from build123d import *

# Parameters (mm, degrees)
SKETCH1_W           = 1
SKETCH1_H           = 18.5735
SKETCH2_R           = 0.7835
BOSS_EXTRUDE1_DEPTH = 0.2165
BOSS_EXTRUDE1_TAPER = -45
SKETCH3_R           = 1
BOSS_EXTRUDE2_DEPTH = 0.222374751
SKETCH4_R           = 1
BOSS_EXTRUDE3_DEPTH = 0.867625249
BOSS_EXTRUDE3_TAPER = -46.049277384
SKETCH5_R           = 1.9
BOSS_EXTRUDE4_DEPTH = 0.12
CUT_EXTRUDE1_DEPTH  = 0.9
CUT_EXTRUDE1_TAPER  = 15
CHAMFER1_SIZE       = 0.2165
FILLET1_R           = 0.5
SCALE1_SCALE        = 3.125


with BuildPart() as part:
    # Sketch1 → Revolve1 (revolve)
    with BuildSketch(Plane.XZ):
        with Locations((0.5, 10.71325)):
            Rectangle(SKETCH1_W, SKETCH1_H)
    revolve(axis=Axis((0, 0, 20), (0, 0, -1)))

    # Sketch2 → Boss-Extrude1 (add)
    with BuildSketch(Plane(origin=(0, 0, 1.4265), x_dir=(-1, 0, 0), z_dir=(0, 0, -1))):
        Circle(SKETCH2_R)
    extrude(amount=BOSS_EXTRUDE1_DEPTH, taper=BOSS_EXTRUDE1_TAPER)

    # Sketch3 → Boss-Extrude2 (add)
    with BuildSketch(Plane(origin=(0, 0, 1.21), x_dir=(-1, 0, 0), z_dir=(0, 0, -1))):
        Circle(SKETCH3_R)
    extrude(amount=BOSS_EXTRUDE2_DEPTH)

    # Sketch4 → Boss-Extrude3 (add)
    with BuildSketch(Plane(origin=(0, 0, 0.987625249), x_dir=(-1, 0, 0), z_dir=(0, 0, -1))):
        Circle(SKETCH4_R)
    extrude(amount=BOSS_EXTRUDE3_DEPTH, taper=BOSS_EXTRUDE3_TAPER)

    # Sketch5 → Boss-Extrude4 (add)
    with BuildSketch(Plane(origin=(0, 0, 0.12), x_dir=(-1, 0, 0), z_dir=(0, 0, -1))):
        Circle(SKETCH5_R)
    extrude(amount=BOSS_EXTRUDE4_DEPTH)

    # Sketch6 → Cut-Extrude1 (cut)
    with BuildSketch(Plane(origin=(0, 0, 0), x_dir=(-1, 0, 0), z_dir=(0, 0, -1))):
        Polygon((-0.95, -0.158333333), (-0.410095116, -0.410095116), (-0.158333333, -0.95), (0.158333333, -0.95), (0.410095116, -0.410095116), (0.95, -0.158333333), (0.95, 0.158333333), (0.410095116, 0.410095116), (0.158333333, 0.95), (-0.158333333, 0.95), (-0.410095116, 0.410095116), (-0.95, 0.158333333), align=None)
    extrude(amount=-CUT_EXTRUDE1_DEPTH, taper=CUT_EXTRUDE1_TAPER, mode=Mode.SUBTRACT)

    # Chamfer1
    chamfer1_edges = [part.edges().sort_by_distance(p)[0] for p in [
        (-1, 0, 20),
    ]]
    chamfer(chamfer1_edges, length=CHAMFER1_SIZE)

    # Fillet1
    fillet1_edges = [part.edges().sort_by_distance(p)[0] for p in [
        (1, 0, 0.987625249),
    ]]
    fillet(fillet1_edges, radius=FILLET1_R)


with BuildPart() as part_1:
    # Scale1: scaled about (8e-09, 0, 9.540596362)
    add(part.part.scale(SCALE1_SCALE).moved(Location((-1.7e-08, 0, -20.273767269))))


solid = part_1.part
Verification items for the finished model (mm, model axes). A direction names the side the tool comes from. Coordinates: 2 decimals unless noted, no trailing zeros. Loops run counter-clockwise (first coordinate to the right, second up) from the corner with the lowest first, then second, coordinate; pieces in that order, holes last. Notation, with made-up numbers: M -17,-16.5 L -4,-16.5 A16 ccw -4,-10.5 Z; hole C -24,-40 d9. An arc over 180 degrees is marked long. One line per item, written item: value.
1. Set-up check for faces 1 (the flat face through (2, 2, -15.816)), 2 (the cylindrical face through (2.98, -0.94, 13.27)), 3 (the cylindrical face through (1.287, -5.796, -20.084)): record each of +Z, -Z, +X, -X, +Y, -Y from which the full face is reachable in a straight line by a thin tool's end or side.
Answers follow:
face 1: none
face 2: +Z
face 3: +Z, -Z
2. Mould release check, pull along X, two halves, no side actions. Record for faces 4 (the conical face through (-3.46, -1.44, -17.79)), 5 (the flat face through (1.4, 1.4, -20.274)), 6 (the flat face through (0, 0, -17.461)): pulls with the +X half, pulls with the -X half, needs draft (parallel to the pull), parting line crosses it, or undercut.
Answers follow:
face 4: parting line crosses it
face 5: needs draft
face 6: undercut
3. Section check A-A on z = -14. Record the cut outline in (x, y) (3 decimals).
Answers follow:
outline: C 0,0 d6.25
4. Material ranges on line 1 along X through (y, z) = (-0.25, 30.5); line 2 along Y through (x, z) = (-1, -1), recorded low to high. Write a range as from..to.
Answers follow:
line 1: -3.11..3.11
line 2: -2.96..2.96
5. Gauge pin test, flat ends, axial feed: P1, Ø3, axis at y = 1, z = 12.5, coming from the +X side (3 decimals); P2, Ø3, axis at y = 0, z = 17, coming from the -X side (3 decimals); P3, Ø2, axis at x = 3.5, z = 35, coming from the -Y side (3 decimals). Record the tip position at first contact, or that the pin passes through.
Answers follow:
P1: x = 3.125
P2: x = -3.125
P3: y = -1.875
